Could you check a few things on this drawing? It's one solid part, dimensions in mm from its lowest x, y, z. A direction names the side the tool comes from. Coordinates: 2 decimals unless noted, no trailing zeros. Order: outer loops, then holes, each group sorted by start corner. A loop starts at its lowest first (then second) coordinate and runs counter-clockwise, first axis right, second up. Notation, with made-up numbers: (30.5, -3) -> (82.5, -3) arc R28 cw to (82.5, 23) -> close; hole circle Ø6 at (-35, 67). An arc over 180 degrees is marked (long way). Use a Markdown table: item, result. Add a question column.
1. If I drill on line 1 along Y through (x, z) = (30, 24); line 2 along Z through (x, y) = (18.25, 30.6); line 3 along Y through (x, z) = (2, 25), over which ranges is the centre line in solid material (lowest first)? Write a range as from..to.
2. Suppose I cut it at D-D, the plane y = 8.5. List the corners of the cut face in (x, z) for me.
3. Suppose I cut it at B-B, the plane x = 18.25. List the corners of the cut face in (y, z) for me.
4. For the marked faces 4 and 5, which set-ups out of +Z, -Z, +X, -X, +Y, -Y let a thin tool reach every point of the face, with its end or its side?
5. Suppose I cut it at C-C, the plane y = 17. List the corners of the cut face in (x, z) for me, then the cut area to 3 significant figures.
6. For pin 1 Ø3 at (x, y) = (25.5, 26) entering from +Z; pin 2 Ø3 at (x, y) = (8, 20) entering from -Z; pin 3 Ø12 at (x, y) = (6.5, 26.5) entering from +Z; pin 4 Ø5 at (x, z) = (20, 27) entering from -Y, each with a flat end and sliding along its axis, tell me the tip position at first contact or that it passes through.
7. Suppose I cut it at A-A, the plane z = 18.25. List the corners of the cut face in (x, y) for me.
8. We'd pull the mould along X, two halves only. Please class the marked faces 1, 2 and 3: pulls with the +X half, pulls with the -X half, needs draft (parallel to the pull), parting line crosses it, or undercut.
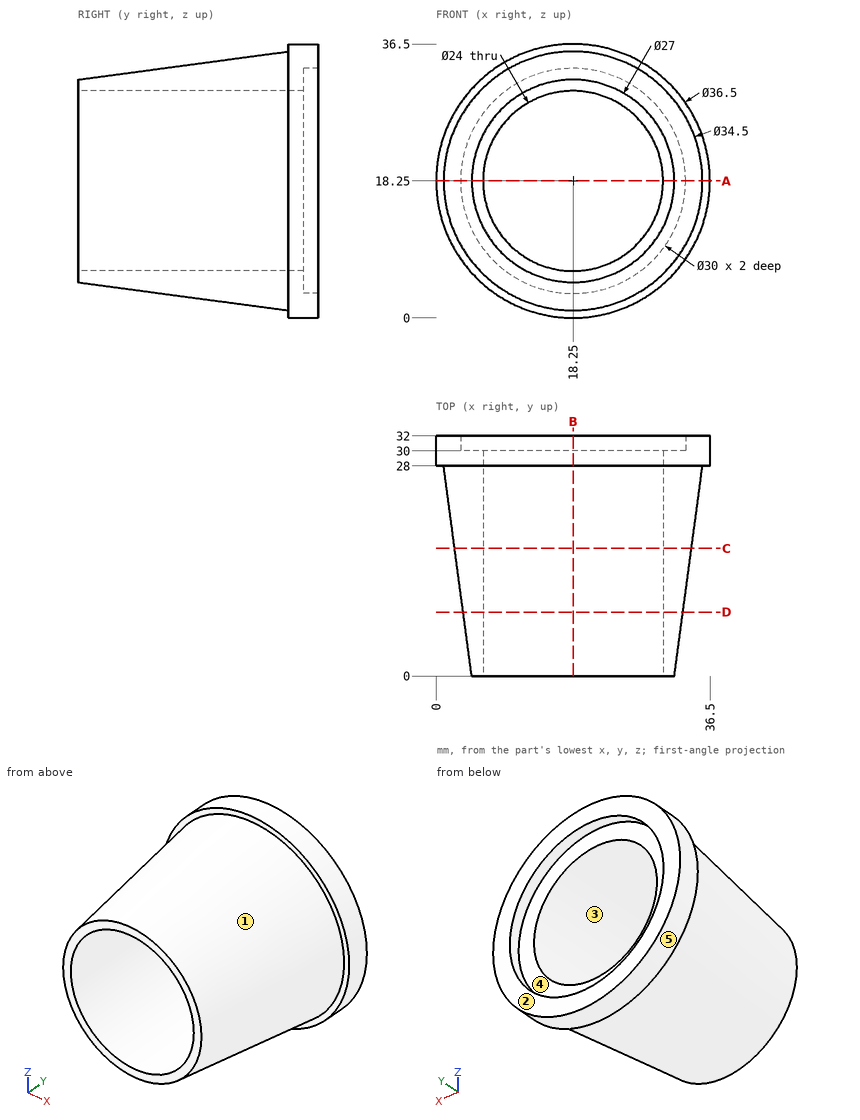
Worked out:
| question | item | result |
|---|---|---|
| 1 | line 1 | y = 0..30 |
| 1 | line 2 | z = 0..3.25, 33.25..36.5 |
| 1 | line 3 | y = 28..32 |
| 2 | outline | circle Ø29.28 at (18.25, 18.25); hole circle Ø24 at (18.25, 18.25) |
| 3 | outline | (0, 4.75) -> (28, 1) -> (28, 0) -> (32, 0) -> (32, 3.25) -> (30, 3.25) -> (30, 6.25) -> (0, 6.25) -> close; (0, 30.25) -> (30, 30.25) -> (30, 33.25) -> (32, 33.25) -> (32, 36.5) -> (28, 36.5) -> (28, 35.5) -> (0, 31.75) -> close |
| 4 | face 4 | +Y |
| 4 | face 5 | +Y, -Y |
| 5 | outline | circle Ø31.55 at (18.25, 18.25); hole circle Ø24 at (18.25, 18.25) |
| 5 | area | 330 mm² |
| 6 | pin 1 | stops at z = 34.27 |
| 6 | pin 2 | stops at z = 4.61 |
| 6 | pin 3 | stops at z = 35.51 |
| 6 | pin 4 | passes through |
| 7 | outline | (0, 28) -> (1, 28) -> (4.75, 0) -> (6.25, 0) -> (6.25, 30) -> (3.25, 30) -> (3.25, 32) -> (0, 32) -> close; (30.25, 0) -> (31.75, 0) -> (35.5, 28) -> (36.5, 28) -> (36.5, 32) -> (33.25, 32) -> (33.25, 30) -> (30.25, 30) -> close |
| 8 | face 1 | parting line crosses it |
| 8 | face 2 | needs draft |
| 8 | face 3 | undercut |
